Part print with two shaded views. Sizes in mm from the minimum x, y, z corner. Give positions to 0.01 mm unless a question says otherwise; leave off trailing zeros. Loops run counter-clockwise (first coordinate to the right, second up) from the corner with the lowest first, then second, coordinate; pieces in that order, holes last. Notation, with made-up numbers: M -24,34 L -18,34 A22 ccw -18,47 Z; hole C 38,56 d4. An arc over 180 degrees is marked long. Answer as a JSON object with one key per item and string values. Group by question number.
1. Slice it at A-A (z = 6). List the corners of the cut face in (x, y).
2. Slice it at C-C (y = 1.45). List the corners of the cut face in (x, z), then the cut area to 3 significant figures.
3. Mould opens along X. For the marked faces 1, 2 and 3 say: released by +X, released by -X, zero draft, split by the parting line, or undercut.
4. Slice it at B-B (x = 6). List the corners of the cut face in (y, z), then the cut area to 3 significant figures.
5. Drill centre lines: line 1 along X through (y, z) = (0.45, 6); line 2 along X through (y, z) = (2.1, 7); line 3 along Z through (x, y) = (4.5, 1.6). Where is each one in solid material? Low to high. Write a range as [from, to].
6. Slice it at D-D (y = 3.55). List the corners of the cut face in (x, z).
7. Drop a flat-ended pin along its axis: pin 1 Ø2.5 at (x, z) = (6, 6) entering from -Y. Give the stop position or say it passes through.
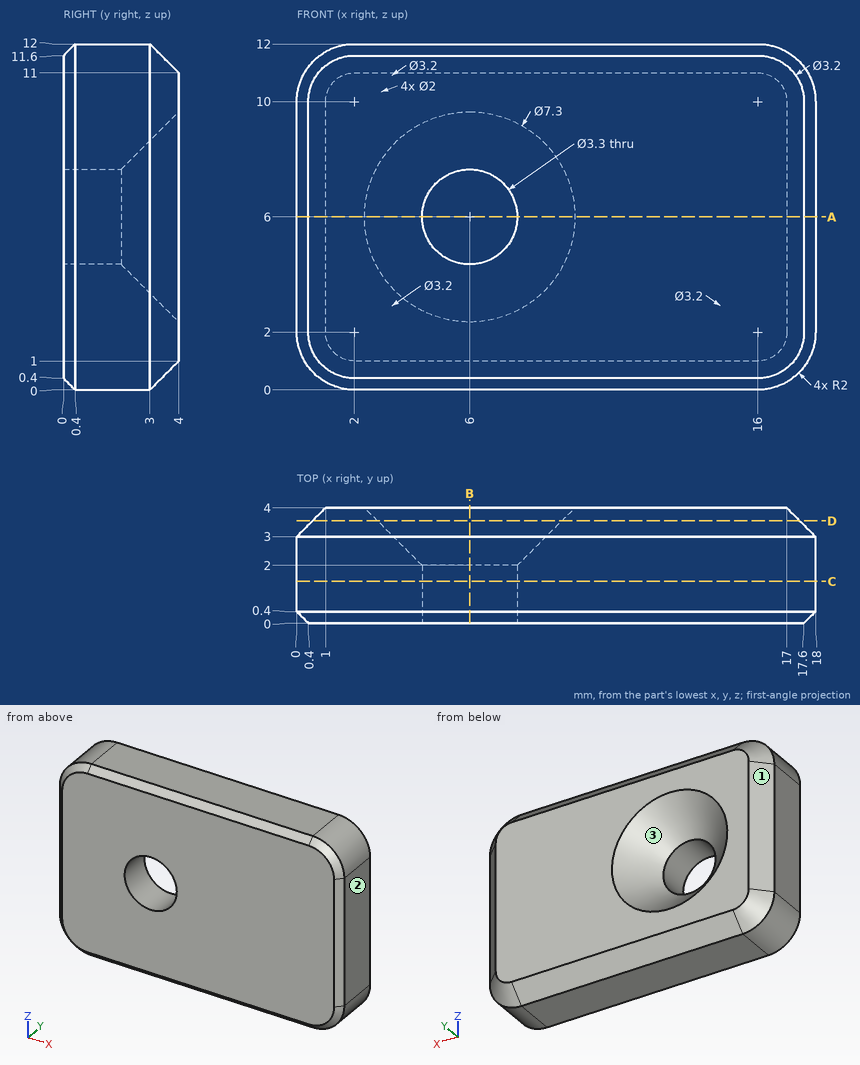
Established:
{
 "1": {"outline": "M 0,0.4 L 0.4,0 L 4.35,0 L 4.35,2 L 2.35,4 L 1,4 L 0,3 Z; M 7.65,0 L 17.6,0 L 18,0.4 L 18,3 L 17,4 L 9.65,4 L 7.65,2 Z"},
 "2": {"outline": "M 0,2 A2 ccw 2,0 L 16,0 A2 ccw 18,2 L 18,10 A2 ccw 16,12 L 2,12 A2 ccw 0,10 Z; hole C 6,6 d3.3", "area": "204 mm^2"},
 "3": {"face 1": "released by -X", "face 2": "released by +X", "face 3": "undercut"},
 "4": {"outline": "M 0,0.4 L 0.4,0 L 3,0 L 4,1 L 4,2.35 L 2,4.35 L 0,4.35 Z; M 0,7.65 L 2,7.65 L 4,9.65 L 4,11 L 3,12 L 0.4,12 L 0,11.6 Z", "area": "29.6 mm^2"},
 "5": {"line 1": "x = [0, 4.35], [7.65, 18]", "line 2": "x = [0, 4.56], [7.44, 18]", "line 3": "z = [0, 5.31], [6.69, 12]"},
 "6": {"outline": "M 0.55,2 A1.45 ccw 2,0.55 L 16,0.55 A1.45 ccw 17.45,2 L 17.45,10 A1.45 ccw 16,11.45 L 2,11.45 A1.45 ccw 0.55,10 Z; hole C 6,6 d6.4"},
 "7": {"pin 1": "passes through"}
}
